The model under review builds one solid part; all positions refer to its coordinate system, in mm. A direction names the side the tool comes from. Give positions to 0.01 mm unless a question says otherwise; leave off trailing zeros. Use CSV: the item, a comma, the result in double quotes.
Autodesk Inventor part; units mm, degrees
ref_plane "YZ Plane" through (0, 0, 0) normal (1, 0, 0) x (0, 1, 0)
ref_plane "XZ Plane" through (0, 0, 0) normal (0, 1, 0) x (-1, 0, 0)
ref_plane "XY Plane" through (0, 0, 0) normal (0, 0, 1) x (1, 0, 0)
sketch "Sketch1" plane through (0, 0, 0) normal (0, 0, 1) x (1, 0, 0)
  line L0 (-2.9393, 4) -> (2.9393, 4)
  line L1 (4, 2.9393) -> (4, -2.9393)
  line L2 (2.9393, -4) -> (-2.9393, -4)
  line L3 (-4, -2.9393) -> (-4, 2.9393)
  line L4 (0, 0) -> (4, -4) construction
  line L5 (-0.5303, -0.5303) -> (-4, -4) construction
  line L6 (5.0607, 4) -> (10, 4) construction
  line L7 (8.2426, 7.182) -> (8.2426, 3.2426)
  line L8 (8.2426, 3.2426) -> (10.2426, 3.2426)
  line L9 (10.2426, 3.2426) -> (10.2426, 10.2426)
  line L10 (10.2426, 10.2426) -> (3.2426, 10.2426)
  line L11 (3.2426, 10.2426) -> (3.2426, 8.2426)
  line L12 (3.2426, 8.2426) -> (7.182, 8.2426)
  line L13 (2.9393, 4) -> (7.182, 8.2426)
  line L14 (4, 2.9393) -> (8.2426, 7.182)
  line L15 (-8.2426, 7.182) -> (-8.2426, 3.2426)
  line L16 (-8.2426, 3.2426) -> (-10.2426, 3.2426)
  line L17 (-10.2426, 3.2426) -> (-10.2426, 10.2426)
  line L18 (-10.2426, 10.2426) -> (-3.2426, 10.2426)
  line L19 (-3.2426, 10.2426) -> (-3.2426, 8.2426)
  line L20 (-3.2426, 8.2426) -> (-7.182, 8.2426)
  line L21 (-2.9393, 4) -> (-7.182, 8.2426)
  line L22 (-4, 2.9393) -> (-8.2426, 7.182)
  line L23 (-2.9393, -4) -> (2.9393, -4)
  line L24 (4, -2.9393) -> (4, 2.9393)
  line L25 (-4, 2.9393) -> (-4, -2.9393)
  line L26 (-4, -4) -> (0, 0) construction
  line L27 (5.0607, -4) -> (10, -4) construction
  line L28 (8.2426, -7.182) -> (8.2426, -3.2426)
  line L29 (8.2426, -3.2426) -> (10.2426, -3.2426)
  line L30 (10.2426, -3.2426) -> (10.2426, -10.2426)
  line L31 (10.2426, -10.2426) -> (3.2426, -10.2426)
  line L32 (3.2426, -10.2426) -> (3.2426, -8.2426)
  line L33 (3.2426, -8.2426) -> (7.182, -8.2426)
  line L34 (2.9393, -4) -> (7.182, -8.2426)
  line L35 (4, -2.9393) -> (8.2426, -7.182)
  line L36 (-3.2426, -10.2426) -> (-3.2426, -8.2426)
  line L37 (-2.9393, -4) -> (-7.182, -8.2426)
  line L38 (-8.2426, -7.182) -> (-8.2426, -3.2426)
  line L39 (-3.2426, -8.2426) -> (-7.182, -8.2426)
  line L40 (-4, -2.9393) -> (-8.2426, -7.182)
  line L41 (-10.2426, -3.2426) -> (-10.2426, -10.2426)
  line L42 (-10.2426, -10.2426) -> (-3.2426, -10.2426)
  line L43 (-8.2426, -3.2426) -> (-10.2426, -3.2426)
  point P0 (0, 0)
  point P1 (-4, 4)
  point P2 (-4, 4)
  dimension "d0" = 8
extrude "Extrusion1" add sketch "Sketch1" along normal mid plane 300
properties part number "front axle"
Q1. Insertion check: pin 1 (1 mm diameter, centred on y = 2.5, z = 23, fed in from +X); pin 2 (3 mm diameter, centred on x = -0.5, z = 51, fed in from +Y); pin 3 (1 mm diameter, centred on x = -6.5, y = -3, fed in from -Z); pin 4 (1.8 mm diameter, centred on x = 0.5, z = -66, fed in from -Y). Each pin has a flat end and moves straight along its axis. Give the tip position at first contact, or say it passes through.
Derived:
pin 1,"stops at x = 4.06"
pin 2,"stops at y = 4"
pin 3,"passes through"
pin 4,"stops at y = -4"
Q2. To check wall thickness, follow probe 1 along X at (y, z) = (8.5, -45); probe 2 along X at (y, z) = (5.25, 38); probe 3 along Y at (x, z) = (5.5, 86). State the ranges of each line that lie inside material, in increasing order.
Derived:
probe 1,"x = -10.24 to -3.24, 3.24 to 10.24"
probe 2,"x = -10.24 to -8.24, -6.31 to -4.19, 4.19 to 6.31, 8.24 to 10.24"
probe 3,"y = -10.24 to -8.24, -6.56 to -4.44, 4.44 to 6.56, 8.24 to 10.24"
Q3. The part is to be moulded in two halves that separate along Y. For faces 4 (the flat face through (4, 0, -2)), 5 (the flat face through (-4, 0, -2)), 6 (the flat face through (7, 10.243, -2)), 7 (the flat face through (-10.243, 7, -2)), say which applies: pulls with the +Y half, pulls with the -Y half, needs draft (parallel to the pull), parting line crosses it, or undercut.
Derived:
face 4,"undercut"
face 5,"undercut"
face 6,"pulls with the +Y half"
face 7,"needs draft"
Q4. Machinability: for faces 1 (the flat face through (0, 4, -2)), 2 (the flat face through (0, -4, -2)), 3 (the flat face through (-7, 10.243, -2)), which of the approach directions +Z, -Z, +X, -X, +Y, -Y give a long, thin tool a straight path to every point of the face, cutting with its end or side? Answer none if there is none.
Derived:
face 1,"+Z, -Z, +Y"
face 2,"+Z, -Z, -Y"
face 3,"+Z, -Z, +X, -X, +Y"
